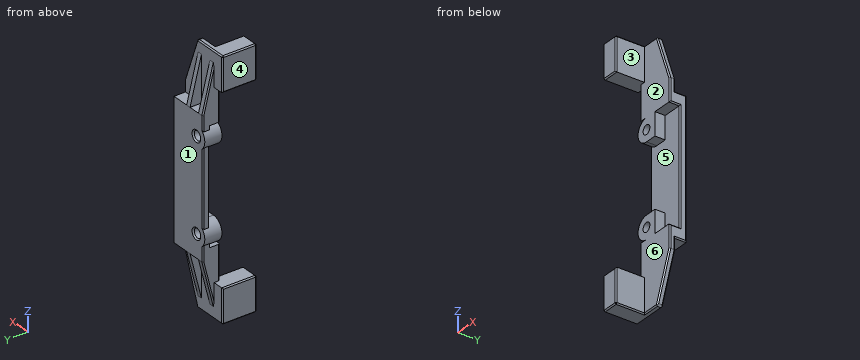
```python
from build123d import *
from OCP.BRepFilletAPI import BRepFilletAPI_MakeChamfer

# Parameters (mm, degrees)
SKETCH_1_W          = 7
SKETCH_1_H          = 44
EXTRUDE_1_DEPTH     = 3
CUT_EXTRUDE_1_DEPTH = 23.477766793
CUT_EXTRUDE_2_DEPTH = 24.280893454
RIB_4_REACH         = 25.281
SKETCH_4_WALL_W     = 56.807998158
SKETCH_4_WALL_H     = 1
RIB_5_REACH         = 24.561
SKETCH_5_WALL_W     = 55.368267942
SKETCH_5_WALL_H     = 0.8
SKETCH_10_W         = 20
SKETCH_10_H         = 3.6
CUT_EXTRUDE_3_DEPTH = 24.280893454
EXTRUDE_2_DEPTH     = 3
EXTRUDE_START       = -1
SKETCH_9_W          = 6
SKETCH_9_H          = 6
EXTRUDE_3_DEPTH     = 3
CHAMFER_1_SIZE      = 0.2
CHAMFER_1_SIZE2     = 0.34176015
CHAMFER_2_SIZE      = 0.2
CHAMFER_3_SIZE      = 0.2


with BuildPart() as part:
    # 草图1 → 凸台-拉伸1 (new body)
    with BuildSketch(Plane(origin=(0, 0, 0), x_dir=(1, 0, 0), z_dir=(0, 1, 0))):
        Rectangle(SKETCH_1_W, SKETCH_1_H)
    extrude(amount=EXTRUDE_1_DEPTH)

    # 草图2 → 切除-拉伸1 (cut, through all)
    with BuildSketch(Plane(origin=(0, 3, 0), x_dir=(1, 0, 0), z_dir=(0, 1, 0))):
        Polygon((3.5, 22), (0.5, 22), (3.5, 14), align=None)
        Polygon((3.5, -22), (0.5, -22), (3.5, -14), align=None)
    extrude(amount=-CUT_EXTRUDE_1_DEPTH, mode=Mode.SUBTRACT)

    # 草图3 → 切除-拉伸2 (cut, through all)
    with BuildSketch(Plane(origin=(3.5, 0, 0), x_dir=(0, 0, -1), z_dir=(1, 0, 0))):
        Polygon((-14, 2.6), (-14, 3), (-22, 3), (-22, 1), align=None)
        Polygon((-14, 1), (-14, 2.6), (-22, 1), align=None)
        Polygon((-12, 1), (-12, 3), (-14, 2.6), (-14, 1), align=None)
        Polygon((-14, 2.6), (-12, 3), (-14, 3), align=None)
        Polygon((14, 2.6), (12, 3), (12, 1), (14, 1), align=None)
        Polygon((22, 1), (14, 2.6), (14, 1), align=None)
        Polygon((22, 3), (14, 3), (14, 2.6), (22, 1), align=None)
        Polygon((14, 3), (12, 3), (14, 2.6), align=None)
    extrude(amount=-CUT_EXTRUDE_2_DEPTH, mode=Mode.SUBTRACT)

    # 草图4 wall → 筋4 (add, up to next)
    with BuildSketch(Plane(origin=(-3.5, 2, 16), x_dir=(0, -0.242535625036, 0.970142500145), z_dir=(0, 0.970142500145, 0.242535625036)), mode=Mode.PRIVATE) as rib_4_sk1:
        with Locations((0, 0.5)):
            Rectangle(SKETCH_4_WALL_W, SKETCH_4_WALL_H)
    rib_4_tool1 = extrude(rib_4_sk1.sketch, amount=-RIB_4_REACH, mode=Mode.PRIVATE) - part.part
    rib_4 = rib_4_tool1.solids().sort_by_distance((-3.5, 2, 16))[0]
    add(rib_4)

    # 草图5 wall → 筋5 (add, up to next)
    with BuildSketch(Plane(origin=(-0.5, 2, 16), x_dir=(0, -0.242535625036, 0.970142500145), z_dir=(0, 0.970142500145, 0.242535625036)), mode=Mode.PRIVATE) as rib_5_sk1:
        with Locations((0, 0.4)):
            Rectangle(SKETCH_5_WALL_W, SKETCH_5_WALL_H)
    rib_5_tool1 = extrude(rib_5_sk1.sketch, amount=-RIB_5_REACH, mode=Mode.PRIVATE) - part.part
    rib_5 = rib_5_tool1.solids().sort_by_distance((-0.5, 2, 16))[0]
    add(rib_5)

    # 草图10 → 切除-拉伸3 (cut, through all)
    with BuildSketch(Plane.ZY.offset(3.5)):
        Rectangle(SKETCH_10_W, SKETCH_10_H)
    extrude(amount=-CUT_EXTRUDE_3_DEPTH, mode=Mode.SUBTRACT)

    # 草图6 → 凸台-拉伸2 (add)
    with BuildSketch(Plane(origin=(0, 3, 0), x_dir=(1, 0, 0), z_dir=(0, 1, 0))):
        with BuildLine():
            Line((0, -6), (-2, -6))
            ThreePointArc((-2, -6), (-4, -8), (-2, -10))
            Line((-2, -10), (0, -10))
            Line((0, -10), (0, -6))
        make_face()
    extrude_2 = extrude(amount=-EXTRUDE_2_DEPTH)

    # 草图8 → M2 螺纹孔1 (revolve, cut)
    with BuildSketch(Plane(origin=(-2, 3, 8), x_dir=(0, 0, 1), z_dir=(1, 0, 0))):
        Polygon((0, 0), (0, 6.480688495), (0.8, 6), (0.8, 0.225), (1.025, 0), align=None)
    hole_wizard_m2_1 = revolve(axis=Axis((-2, 9.35, 8), (0, -1, 0)), mode=Mode.SUBTRACT)

    # 草图9 → 凸台-拉伸3 (add)
    with BuildSketch(Plane.ZY.offset(3.5).offset(EXTRUDE_START)):
        with Locations((19, -2)):
            Rectangle(SKETCH_9_W, SKETCH_9_H)
    extrude_3 = extrude(amount=EXTRUDE_3_DEPTH)

    # 镜向1: 筋4, 筋5, 凸台-拉伸2, M2 螺纹孔1, 凸台-拉伸3 across plane
    add(rib_4.mirror(Plane.XY))
    add(rib_5.mirror(Plane.XY))
    add(extrude_2.mirror(Plane.XY))
    add(hole_wizard_m2_1.mirror(Plane.XY), mode=Mode.SUBTRACT)
    add(extrude_3.mirror(Plane.XY))

    # 倒角1: one chamfer whose edges measure the first distance from different faces: ONE call of the kernel's chamfer builder (chamfer() names one face for all edges)
    chamfer_1_edges_1 = [part.edges().sort_by_distance(p)[0] for p in [
        (0.5, 0.5, -22),
    ]]
    chamfer_1_side_1 = [part.faces().sort_by_distance(p)[0] for p in [
        (-3.571428571, -1.642857143, -22),
    ]]
    chamfer_1_edges_2 = [part.edges().sort_by_distance(p)[0] for p in [
        (-1, 0, 22),
        (-2.5, -2.5, 22),
        (-4, -5, 22),
        (-2.5, -5, 19),
        (-4, -5, 16),
        (-5.5, -2, 22),
        (-5.5, 1, 19),
        (-5.5, -2, 16),
        (-5.5, -5, 19),
        (-1, 0, -22),
        (-4, -5, -22),
        (-5.5, -2, -22),
        (-5.5, -2, -16),
        (-5.5, 1, -19),
        (-4, -5, -16),
        (-5.5, -5, -19),
        (-2.5, -2.5, -22),
        (-2.5, -5, -19),
        (-2.5, 1, 22),
        (-2.5, 1, -22),
    ]]
    chamfer_1_edges_3 = [part.edges().sort_by_distance(p)[0] for p in [
        (0.5, 0.5, 22),
    ]]
    chamfer_1_side_3 = [part.faces().sort_by_distance(p)[0] for p in [
        (2, 0.5, 18),
    ]]
    chamfer_1 = BRepFilletAPI_MakeChamfer(part.part.solid().wrapped)
    for e in chamfer_1_edges_1:
        chamfer_1.Add(CHAMFER_1_SIZE, CHAMFER_1_SIZE2, e.wrapped, chamfer_1_side_1[0].wrapped)  # the first distance lies on this face
    for e in chamfer_1_edges_2:
        chamfer_1.Add(CHAMFER_1_SIZE, e.wrapped)
    for e in chamfer_1_edges_3:
        chamfer_1.Add(CHAMFER_1_SIZE, CHAMFER_1_SIZE2, e.wrapped, chamfer_1_side_3[0].wrapped)  # the first distance lies on this face
    add(Compound.cast(chamfer_1.Shape()), mode=Mode.REPLACE)

    # 倒角2
    chamfer_2_edges = [part.edges().sort_by_distance(p)[0] for p in [
        (2.06, 0, -17.84),
        (2.06, 1, -17.84),
        (3.5, 0, -12),
        (3.5, 0.9, -10),
        (3.5, 1.8, 0),
        (3.5, 0.9, 10),
        (3.5, 0, 12),
        (2.0375, 0, 17.9),
        (3.5, 1, -13),
        (3.5, 2, -12),
        (3.5, 3, 0),
        (3.5, 2, 12),
        (3.5, 1, 13),
        (2.0375, 1, 17.9),
    ]]
    chamfer(chamfer_2_edges, length=CHAMFER_2_SIZE)

    # 倒角3
    chamfer_3_edges = [part.edges().sort_by_distance(p)[0] for p in [
        (-3.5, 0, 13),
        (-3.5, 1.8, 0),
        (-3.5, 3, 10.661437828),
        (-3.5, 2, -16),
        (-3.5, 3, 0),
        (-3.5, 0, -13),
        (-3.5, 3, -10.661437828),
        (-3.5, 2, 16),
    ]]
    chamfer(chamfer_3_edges, length=CHAMFER_3_SIZE)


solid = part.part
```
Can you work these out from the model? Positions are in its coordinate system, mm. Face numbers are marked on the shaded views. A direction names the side the tool comes from. Round coordinates to 2 decimals unless told otherwise and drop trailing zeros. Order: outer loops, then holes, each group sorted by start corner. A loop starts at its lowest first (then second) coordinate and runs counter-clockwise, first axis right, second up.
(1) If we section it at D-D (x = 1): Please give me the cut outline in (y, z).
Results are:
outline: (0, -20.1) - (0.2, -20.67) - (0.8, -20.67) - (1, -20.1) - (1, -12) - (3, -12) - (3, 12) - (1, 12) - (1, 20.1) - (0.8, 20.67) - (0.2, 20.67) - (0, 20.1) - (0, 10) - (1.8, 10) - (1.8, -10) - (0, -10) - close
(2) We'd pull the mould along Z, two halves only. Please class the marked faces 4, 5 and 6: +Z half, -Z half, draft (parallel to the pull), parting line (faces both ways), or undercut.
Results are:
face 4: draft
face 5: undercut
face 6: undercut
(3) If I drill on L1, parallel to X at y = 1.5, z = 8; L2, parallel to Y at x = 3, z = -3; L3, parallel to Z at x = -3.5, y = -4.25, over which ranges is the centre line in solid material (lowest first)?
Results are:
L1: x = -4 to -2.8, -1.2 to 0
L2: y = 1.8 to 3
L3: z = -22 to -16, 16 to 22
(4) If we section it at A-A (y = -3.5): Please give me the cut outline in (x, z).
Results are:
outline: (-5.5, -21.8) - (-5.3, -22) - (-2.7, -22) - (-2.5, -21.8) - (-2.5, -16) - (-5.3, -16) - (-5.5, -16.2) - close; (-5.5, 16.2) - (-5.3, 16) - (-2.5, 16) - (-2.5, 21.8) - (-2.7, 22) - (-5.3, 22) - (-5.5, 21.8) - close
(5) If we section it at B-B (z = -8): Please give me the cut outline in (x, y) (3 decimals).
Results are:
outline: (-4, 0) - (-2.8, 0) - (-2.8, 2.775) - (-3.025, 3) - (-4, 3) - close; (-1.2, 0) - (0, 0) - (0, 1.8) - (3.3, 1.8) - (3.5, 2) - (3.5, 2.8) - (3.3, 3) - (-0.975, 3) - (-1.2, 2.775) - close
(6) I'm going to push flat-ended pins straight in: pin 1 (2 mm diameter, centred on x = -4, z = 1.5, fed in from +Y); pin 2 (4 mm diameter, centred on x = 0.5, z = 7, fed in from -Y); pin 3 (1.6 mm diameter, centred on y = 2, z = -15.5, fed in from -X); pin 4 (1.3 mm diameter, centred on x = -2, z = 8, fed in from -Y). Where does each tip first touch, or does it pass through?
Results are:
pin 1: stops at y = 3
pin 2: stops at y = 0
pin 3: stops at x = -3.5
pin 4: passes through
(7) On a 3-axis mill with a long thin cutter (end or side, diameter ignored), from which of +Z, -Z, +X, -X, +Y, -Y can I reach the whole of each face in a straight line? I mean the marked faces 1, 2 and 3. Say none if no direction works.
Results are:
face 1: +Z, -Z, +X, -X, +Y
face 2: +X, -Y
face 3: +Z, -Z, +X, -Y
(8) If we section it at C-C (z = 11): Please give me the cut outline in (x, y).
Results are:
outline: (-3.5, 0.2) - (-3.3, 0) - (3.3, 0) - (3.5, 0.2) - (3.5, 2.8) - (3.3, 3) - (-3.3, 3) - (-3.5, 2.8) - close
